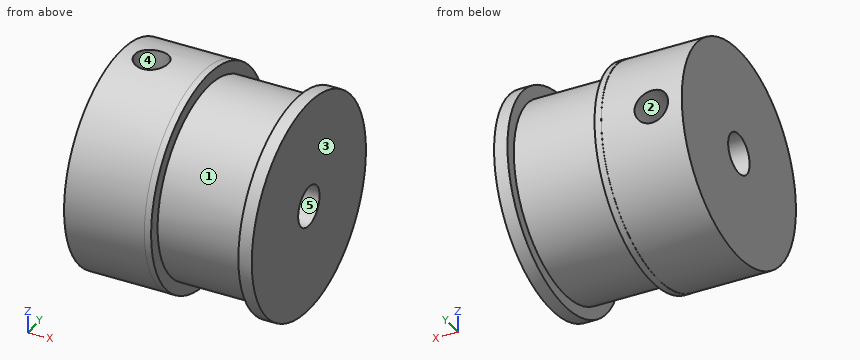
```python
from build123d import *

# Parameters (mm, degrees)
SKETCH2_W = 1.25
SKETCH2_H = 8.015739734
SKETCH4_W = 1.25
SKETCH4_H = 8.015739734


with BuildPart() as part:
    # Sketch1 → Revolve1 (revolve)
    with BuildSketch(Plane.XY):
        Polygon((1.451473536, 1.5), (1.451473536, 8), (7.451473536, 8), (7.451473536, 8.015739734), (7.951473536, 8.015739734), (7.951473536, 7.104033654), (14.451473536, 7.104033654), (14.451473536, 8), (15.451473536, 8), (15.451473536, 1.5), align=None)
    revolve(axis=Axis((0, 0, 0), (-1, 0, 0)))

    # Sketch2 → M3x0.5 Tapped Hole1 (revolve, cut)
    with BuildSketch(Plane(origin=(3.725736768, 0, 0), x_dir=(0, 0, -1), z_dir=(1, 0, 0))):
        with Locations((0.625, 4.007869867)):
            Rectangle(SKETCH2_W, SKETCH2_H)
    revolve(axis=Axis((3.725736768, -6.35, 0), (0, 1, 0)), mode=Mode.SUBTRACT)

    # Sketch4 → M3x0.5 Tapped Hole2 (revolve, cut)
    with BuildSketch(Plane.YZ.offset(3.725736768)):
        with Locations((0.625, 4.007869867)):
            Rectangle(SKETCH4_W, SKETCH4_H)
    revolve(axis=Axis((3.725736768, 0, -6.35), (0, 0, 1)), mode=Mode.SUBTRACT)


solid = part.part
```
The model under review builds one solid part; all positions refer to its coordinate system, in mm. Face numbers are marked on the shaded views. A direction names the side the tool comes from. Round coordinates to 2 decimals unless told otherwise and drop trailing zeros. Write each loop counter-clockwise with the first axis right and the second up, starting at its lowest first coordinate (ties: lowest second). Pieces come first, ordered by that corner, then holes.
(1) Insertion check: pin 1 (2 mm diameter, centred on x = 3.73, z = 0, fed in from -Y); pin 2 (2 mm diameter, centred on x = 3.73, y = 0, fed in from -Z); pin 3 (3 mm diameter, centred on x = 4, z = -0.5, fed in from +Y). Each pin has a flat end and moves straight along its axis. Give the tip position at first contact, or say it passes through.
(2) Machinability: for the marked faces 4 and 5, which of the approach directions +Z, -Z, +X, -X, +Y, -Y give a long, thin tool a straight path to every point of the face, cutting with its end or side? Answer none if there is none.
(3) Wall thickness on L1, parallel to X at y = 0, z = 4.75; L2, parallel to X at y = 5.5, z = -5.25; L3, parallel to Y at x = 11.25, z = 0: over which ranges is each line inside the solid? List them lowest first.
(4) Mouldability with a two-part tool opening along Z and no side actions: class the marked faces 1, 2 and 3 as +Z half, -Z half, draft (parallel to the pull), parting line (faces both ways), or undercut.
(5) We need section A-A on z = 0. Give the number of separate pieces and of enclosed holes in the cut face, and give its area (3 significant figures).
(6) We need section D-D on x = 10.25. Give the boundary of the cut face in (y, z).
Findings below:
1. pin 1: stops at y = -8
1. pin 2: stops at z = -8
1. pin 3: stops at y = 8
2. face 4: +Z
2. face 5: +X, -X
3. L1: x = 1.45 to 2.48, 4.98 to 15.45
3. L2: x = 1.45 to 7.95, 14.45 to 15.45
3. L3: y = -7.1 to -1.5, 1.5 to 7.1
4. face 1: parting line
4. face 2: undercut
4. face 3: draft
5. separate pieces: 3
5. enclosed holes: 0
5. area: 154 mm2
6. outline: circle Ø14.21 at (0, 0); hole circle Ø3 at (0, 0)
